Autodesk Inventor part; units mm, degrees
ref_plane "YZ Plane" through (0, 0, 0) normal (1, 0, 0) x (0, 1, 0)
ref_plane "XZ Plane" through (0, 0, 0) normal (0, 1, 0) x (-1, 0, 0)
ref_plane "XY Plane" through (0, 0, 0) normal (0, 0, 1) x (1, 0, 0)
ref_plane "Work Plane1" through (0, 0, 0) normal (0, 0, 1) x (1, 0, 0)
sketch "Sketch1" plane through (0, 0, 0) normal (0, 0, 1) x (1, 0, 0)
  circle A0 centre (0, 0) radius 7.5
  line L0 (-30, 28) -> (-28, 30)
  line L1 (-30, -28) -> (-30, 28)
  line L2 (-28, -30) -> (-30, -28)
  line L3 (28, -30) -> (-28, -30)
  line L4 (30, -28) -> (28, -30)
  line L5 (30, 28) -> (30, -28)
  line L6 (28, 30) -> (30, 28)
  line L7 (-28, 30) -> (28, 30)
  circle A1 centre (25, 25) radius 2.325
  circle A2 centre (-25, -25) radius 2.325
  circle A3 centre (25, -25) radius 2.325
  circle A4 centre (-25, 25) radius 2.325
  point P0 (0, 0)
extrude "Extrusion1" add sketch "Sketch1" along normal blind 18.5 contours A0 | L0 L7 L6 L5 L4 L3 L2 L1 | A1 | A2 | A3 | A4
sketch "Sketch2" plane through (0, 0, 18.5) normal (0, 0, 1) x (1, 0, 0)
  point P0 (0, 0)
sketch "Sketch3" plane through (30, -28, 0) normal (1, 0, 0) x (0, 0, -1)
  line L0 (0, 56) -> (0, 0)
  line L1 (0, 56) -> (-18.5, 56)
  line L2 (-18.5, 0) -> (-18.5, 56)
  line L3 (0, 0) -> (-18.5, 0)
  line L4 (-18.5, 0) -> (-18.5, 56)
  line L5 (0, 47.2331) -> (-18.5, 47.2331)
  line L6 (-18.5, 47.2331) -> (-18.5, 36.3051)
  line L7 (-18.5, 36.3051) -> (0, 36.3051)
  line L8 (0, 36.3051) -> (0, 47.2331)
  line L9 (0, 56) -> (0, 0)
  line L10 (0, 10.2066) -> (-18.5, 10.2066)
  line L11 (-18.5, 10.2066) -> (-18.5, 18.9489)
  line L12 (-18.5, 18.9489) -> (0, 18.9489)
  line L13 (0, 18.9489) -> (0, 10.2066)
  point P0 (0, 28)
extrude "Extrusion2" [suppressed]
sketch "Sketch4" plane through (30, 19.2331, 16) normal (0, 1, 0) x (1, 0, 0)
  line L0 (0, 0) -> (0, 16)
  line L1 (0, 0) -> (14, 0)
  line L2 (14, 16) -> (14, 0)
  line L3 (0, 16) -> (14, 16)
  circle A0 centre (7, 5) radius 1.5
  point P0 (-30, 16)
  dimension "d4" = 3
extrude "Extrusion3" [suppressed]
pattern_circular "Circular Pattern1" [suppressed]
sketch "Sketch5" plane through (-30, -28, 0) normal (-1, 0, 0) x (0, 0, 1)
  circle A0 centre (12.5, 43) radius 1.5
  line L0 (18.5, 56) -> (18.5, 0)
  line L1 (0, 58) -> (18.5, 58)
  circle A1 centre (12.5, 13) radius 2
  line L2 (0, -2) -> (18.5, -2)
  point P0 (0, 28)
  dimension "d10" = 3
  dimension "d11" = 6
  dimension "d12" = 15
  dimension "d13" = 4
  dimension "d14" = 6
  dimension "d15" = 15
extrude "Extrusion4" cut sketch "Sketch5" against normal blind 18.5
pattern_circular "Circular Pattern2" count 4 over 360 about axis through (0, 0, 0) along (0, 0, 1) of "Extrusion4"
properties part number "00_XY_stage-CHUO_SEIKI_LD-647-R1-Middle"
CAD build for the part. Positions are in the model's coordinates, mm. A direction names the side the tool comes from. Round coordinates to 2 decimals unless told otherwise and drop trailing zeros. Loops run counter-clockwise (first coordinate to the right, second up) from the corner with the lowest first, then second, coordinate; pieces in that order, holes last. Notation, with made-up numbers: M 15,67 L 66,67 A22 ccw 66,97 Z; hole C 26,15.25 d10. An arc over 180 degrees is marked long. Return JSON: item names as keys, results as strings. Group by question number.
(1) Saw through at A-A, the plane x = -15. List the corners of the cut face in (y, z).
(2) Tool access for faces 4 (the flat face through (-15, 11.5, 12)), 5 (the flat face through (-11.5, 15, 12)), 6 (the cylindrical face through (14.912, -20.88, 10.502)): list every direction of +Z, -Z, +X, -X, +Y, -Y with a clear straight run to the whole face (end or side of a thin tool).
(3) Wall check: probe 1 along X at (y, z) = (-21.5, 12.5); probe 2 along Y at (x, z) = (-11.95, 12.5). Give the ranges that are in metal, low to high. Write a range as [from, to].
(4) Mould opens along Y. For faces 1 (the flat face through (-11.5, -15, 12)), 2 (the flat face through (15, 11.5, 12)), 3 (the flat face through (-30, 0, 9)) say: +Y half, -Y half, draft (parallel to the pull), parting line (faces both ways), or undercut.
(5) Saw through at D-D, the plane x = -24. List the corners of the cut face in (y, z).
(6) Drop flat-ended pins along their axis: P1, Ø1.5, axis at x = -15.5, z = 12, coming from the -Y side; P2, Ø2.5, axis at x = 14.5, z = 13, coming from the +Y side; P3, Ø2.5, axis at y = 15, z = 12.5, coming from the +X side; P4, Ø3.5, axis at x = -15, z = 12.5, coming from the +Y side. Give the stop position or say it passes through.
(7) Saw through at C-C, the plane z = 12.5. Give the number of separate pieces and of enclosed holes in the cut face, and give its area (3 significant figures).
Answer list:
{
 "1": {"outline": "M -30,0 L 30,0 L 30,10.5 L 11.5,10.5 L 11.5,14.5 L 30,14.5 L 30,18.5 L -30,18.5 L -30,14 L -16.32,14 A2 cw -13.68,14 L -11.5,14 L -11.5,11 L -13.68,11 A2 cw -16.32,11 L -30,11 Z"},
 "2": {"face 4": "+Y", "face 5": "-X", "face 6": "-Y"},
 "3": {"probe 1": "[-30, -16.5], [-13.5, 13], [17, 30]", "probe 2": "[-30, -17], [-13, 13.5], [16.5, 30]"},
 "4": {"face 1": "undercut", "face 2": "+Y half", "face 3": "draft"},
 "5": {"outline": "M -30,0 L 30,0 L 30,18.5 L -30,18.5 Z; hole C -15,12.5 d4; hole C 15,12.5 d3"},
 "6": {"P1": "y = -11.5", "P2": "y = 30", "P3": "x = 11.5", "P4": "y = 11.5"},
 "7": {"separate pieces": "5", "enclosed holes": "0", "area": "3,120 mm2"}
}
